The model under review builds one solid part; all positions refer to its coordinate system, in mm. A direction names the side the tool comes from. Coordinates: 2 decimals unless noted, no trailing zeros. Write each loop counter-clockwise with the first axis right and the second up, starting at its lowest first coordinate (ties: lowest second). Pieces come first, ordered by that corner, then holes. Notation, with made-up numbers: (60, -10) -> (73, -10) arc R29 ccw to (73, 19) -> close; hole circle Ø1 at (12, 83.25). An arc over 180 degrees is marked (long way). Write each question's results on one line, items separated by ' | '.
Autodesk Inventor part; units mm, degrees
ref_plane "YZ Plane" through (0, 0, 0) normal (1, 0, 0) x (0, 1, 0)
ref_plane "XZ Plane" through (0, 0, 0) normal (0, 1, 0) x (-1, 0, 0)
ref_plane "XY Plane" through (0, 0, 0) normal (0, 0, 1) x (1, 0, 0)
sketch "Sketch1" plane through (0, 0, 0) normal (1, 0, 0) x (0, 1, 0)
  line L0 (720, 0) -> (0, -502.4464)
  line L1 (0, -600) -> (720, -97.5536)
  line L2 (0, 0) -> (720, -502.4464)
  line L3 (720, -600) -> (0, -97.5536)
  line L4 (720, 0) -> (720, -97.5536)
  line L5 (720, -502.4464) -> (720, -600)
  line L6 (0, -600) -> (0, -502.4464)
  line L7 (0, -97.5536) -> (0, 0)
  dimension "d0" = 600
  dimension "d1" = 720
  dimension "d2" = 80
  dimension "d3" = 80
sketch "Sketch2" plane through (0, 0, 0) normal (1, 0, 0) x (0, 1, 0)
  point P0 (0, 0)
extrude "Extrusion1" add sketch "Sketch1" along normal blind 80
fillet "Fillet1" radius 5 1 edges at (40, 360, -251.2232)
fillet "Fillet2" radius 5 1 edges at (40, 429.8966, -300)
fillet "Fillet3" radius 5 1 edges at (40, 360, -348.7768)
fillet "Fillet4" radius 5 1 edges at (40, 290.1034, -300)
sketch "Sketch3" plane through (80, 0, 0) normal (1, 0, 0) x (0, 0, -1)
  line L0 (502.4464, 720) -> (600, 720)
  line L1 (0, 723) -> (600, 723)
  line L2 (600, 723) -> (600, 720)
  line L3 (600, 720) -> (0, 720)
  line L4 (0, 720) -> (0, 723)
  point P0 (0, 0)
  dimension "d10" = 600
  dimension "d11" = 3
extrude "Extrusion2" add sketch "Sketch3" against normal blind 80
fillet "Fillet5" radius 5 1 edges at (40, 0, 0)
fillet "Fillet6" radius 5 1 edges at (40, 723, 0)
fillet "Fillet7" radius 5 1 edges at (40, 723, -600)
fillet "Fillet8" radius 5 1 edges at (40, 0, -600)
properties part number "leg" material "Steel"
Q1. Draft analysis for pull direction Y (two halves, no side actions). For faces 1 (the flat face through (39.44, 144.103, -198.115)), 2 (the flat face through (0, 363, -321)), 3 (the flat face through (39.44, 543.93, -477.13)), state which applies: pulls with the +Y half, pulls with the -Y half, needs draft (parallel to the pull), parting line crosses it, or undercut.
Solution:
face 1: pulls with the -Y half | face 2: needs draft | face 3: undercut
Q2. Add section D-D (z = -283). Write out the cut boundary in (x, y), plus the area to 3 significant figures.
Solution:
outline: (0, 265.74) -> (80, 265.74) -> (80, 454.26) -> (0, 454.26) -> close; (0, 720) -> (80, 720) -> (80, 723) -> (0, 723) -> close | area: 15,300 mm²
Q3. Add section C-C (y = 49). Write out the cut boundary in (x, z).
Solution:
outline: (0, -565.81) -> (80, -565.81) -> (80, -468.25) -> (0, -468.25) -> close; (0, -131.75) -> (80, -131.75) -> (80, -34.19) -> (0, -34.19) -> close
Q4. Clearance check with flat-ended pins moving along their axes: P1, Ø2, axis at x = 32.5, y = 336.5, coming from the +Z side; P2, Ø3, axis at y = 513.5, z = -388, coming from the -X side; P3, Ø4, axis at x = 30, z = -246, coming from the -Y side; P4, Ø3, axis at x = 21.5, y = 515, coming from the -Z side. State where each tip first meets the part, or that it passes through.
Solution:
P1: z = -234.13 | P2: x = 0 | P3: y = 209.86 | P4: z = -457.99
Q5. Add section B-B (x = 57). Write out the cut boundary in (y, z), plus the area to 3 significant figures.
Solution:
outline: (0, -590.41) arc R5 ccw to (7.86, -594.51) -> (357.14, -350.77) arc R5 cw to (362.86, -350.77) -> (720, -600) arc R5 ccw to (723, -595.42) -> (723, -4.58) arc R5 ccw to (720, 0) -> (362.86, -249.23) arc R5 cw to (357.14, -249.23) -> (7.86, -5.49) arc R5 ccw to (0, -9.59) -> (0, -97.55) -> (284.23, -295.9) arc R5 cw to (284.23, -304.1) -> (0, -502.45) -> close; hole (435.77, -304.1) -> (720, -502.45) -> (720, -97.55) -> (435.77, -295.9) arc R5 ccw to start | area: 135,000 mm²
Q6. For line 1 (Y direction, x = 7.5, z = -434); line 2 (Y direction, x = 48, z = -192.5); line 3 (Y direction, x = 47, z = -294.5), list the stretches that pass through material, from the lowest coordinate up. Write a range as from..to.
Solution:
line 1: 98.08..237.88, 482.12..621.92, 720..723 | line 2: 136.06..275.85, 444.15..583.94, 720..723 | line 3: 282.22..437.78, 720..723
Q7. Machinability: for faces 4 (the flat face through (39.44, 144.103, -401.885)), 5 (the flat face through (39.44, 543.93, -122.87)), 6 (the flat face through (39.44, 180.055, -474.35)), 7 (the flat face through (41, 723, -296)), 8 (the flat face through (39.44, 575.897, -198.115)), which of the approach directions +Z, -Z, +X, -X, +Y, -Y give a long, thin tool a straight path to every point of the face, cutting with its end or side? Answer none if there is none.
Solution:
face 4: +X, -X, -Y | face 5: +Z, +X, -X | face 6: -Z, +X, -X | face 7: +Z, -Z, +X, -X, +Y | face 8: +X, -X
Q8. Add section A-A (z = -469.5). Write out the cut boundary in (x, y), plus the area to 3 significant figures.
Solution:
outline: (0, 47.21) -> (80, 47.21) -> (80, 187.01) -> (0, 187.01) -> close; (0, 532.99) -> (80, 532.99) -> (80, 672.79) -> (0, 672.79) -> close; (0, 720) -> (80, 720) -> (80, 723) -> (0, 723) -> close | area: 22,600 mm²
